Design review of the part shown in the three views and the two pictorial views. Dimensions are in mm from the part's minimum x, y and z. A direction names the side the tool comes from. Round coordinates to 2 decimals unless told otherwise and drop trailing zeros. Loops run counter-clockwise (first coordinate to the right, second up) from the corner with the lowest first, then second, coordinate; pieces in that order, holes last. Notation, with made-up numbers: M 4,13 L 29,13 A13 cw 29,21 Z; hole C 12,-19.5 d7. An arc over 180 degrees is marked long. Answer in a Markdown table with one row per item. Add a question column.
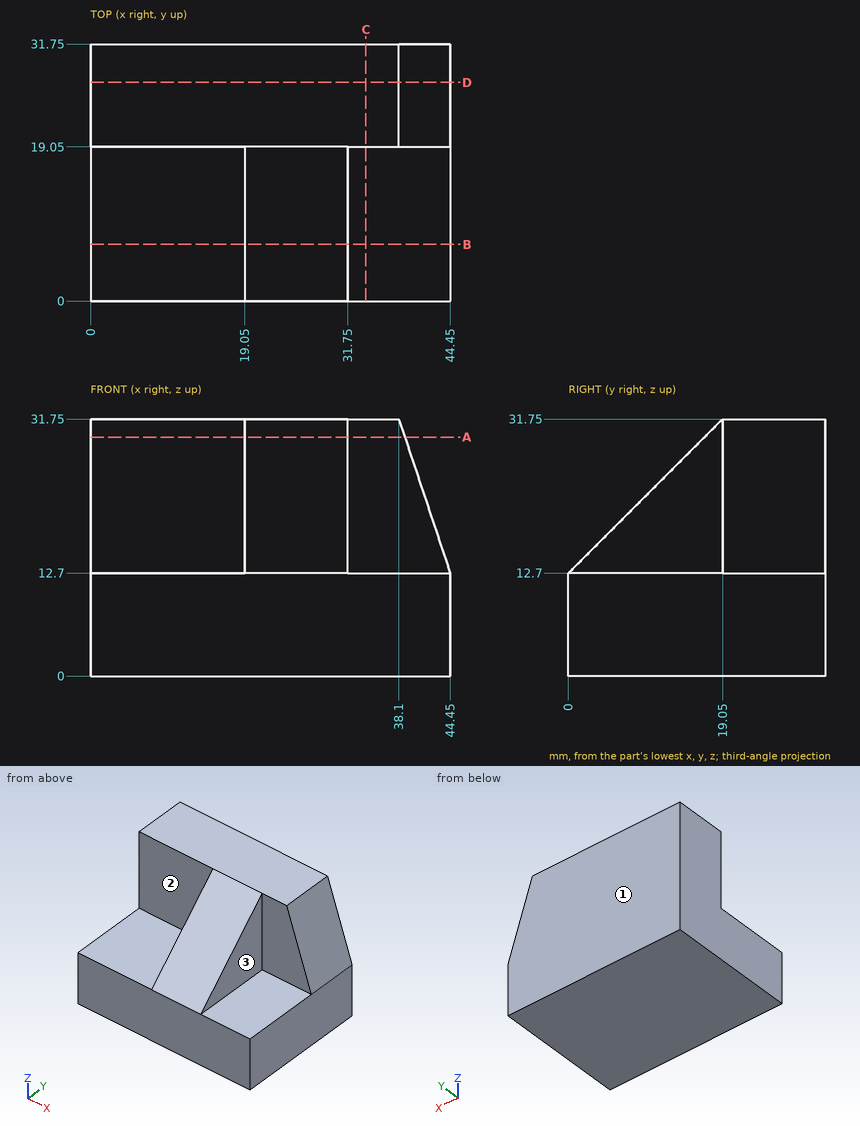
1. To check wall thickness, follow probe 1 along Y at (x, z) = (6, 15); probe 2 along Z at (x, y) = (41, 2). State the ranges of each line that lie inside material, in increasing order.
2. Take a section at A-A, the plane z = 29.5. State the section outline as (x, y) points.
3. Machinability: for the marked faces 1, 2 and 3, which of the approach directions +Z, -Z, +X, -X, +Y, -Y give a long, thin tool a straight path to every point of the face, cutting with its end or side? Answer none if there is none.
4. Take a section at B-B, the plane y = 7. State the section outline as (x, z) points.
5. Take a section at D-D, the plane y = 27. State the section outline as (x, z) points.
6. For pin 1 Ø5.5 at (y, z) = (10, 18) entering from -X; pin 2 Ø5.5 at (y, z) = (14, 26) entering from +X; pin 3 Ø4 at (x, z) = (29.5, 17.5) entering from -Y, all flat-tipped, find the tip position at first contact; note any pin that passes through.
7. Take a section at C-C, the plane x = 34. State the section outline as (y, z) points.
Check sheet entries:
| question | item | result |
|---|---|---|
| 1 | probe 1 | y = 19.05 to 31.75 |
| 1 | probe 2 | z = 0 to 12.7 |
| 2 | outline | M 0,19.05 L 19.05,19.05 L 19.05,16.8 L 31.75,16.8 L 31.75,19.05 L 38.85,19.05 L 38.85,31.75 L 0,31.75 Z |
| 3 | face 1 | +Z, -Z, +X, -X, +Y |
| 3 | face 2 | +Z, -X, -Y |
| 3 | face 3 | +Z, +X, -Y |
| 4 | outline | M 0,0 L 44.45,0 L 44.45,12.7 L 31.75,12.7 L 31.75,19.7 L 19.05,19.7 L 19.05,12.7 L 0,12.7 Z |
| 5 | outline | M 0,0 L 44.45,0 L 44.45,12.7 L 38.1,31.75 L 0,31.75 Z |
| 6 | pin 1 | stops at x = 19.05 |
| 6 | pin 2 | stops at x = 31.75 |
| 6 | pin 3 | stops at y = 2.8 |
| 7 | outline | M 0,0 L 31.75,0 L 31.75,31.75 L 19.05,31.75 L 19.05,12.7 L 0,12.7 Z |
